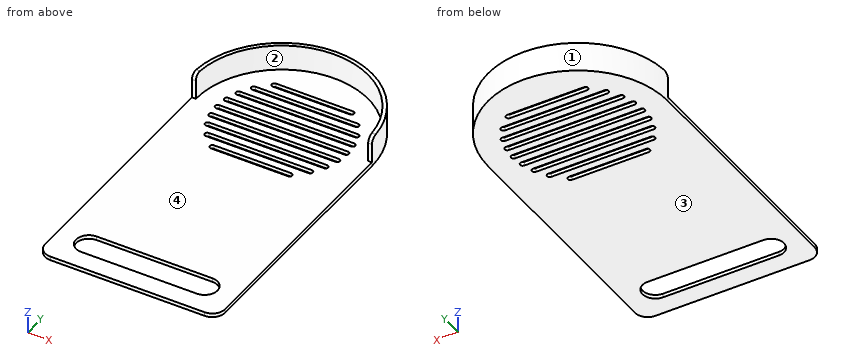
```python
from build123d import *

# Parameters (mm, degrees)
F1_DEPTH = 3
F2_DEPTH = 20
F3_R     = 5


with BuildPart() as f1:
    # F0 (on Top) → F1 (new body)
    with BuildSketch(Plane.XY):
        with BuildLine():
            Line((70, -190), (70, 0))
            Line((70, 0), (67, 0))
            ThreePointArc((67, 0), (0, 67), (-67, 0))
            Line((-67, 0), (-70, 0))
            Line((-70, 0), (-70, -190))
            ThreePointArc((-70, -190), (-67.071068, -197.071068), (-60, -200))
            Line((-60, -200), (60, -200))
            ThreePointArc((60, -200), (67.071068, -197.071068), (70, -190))
        make_face()
        with BuildLine():
            Line((45, -185), (-45, -185))
            ThreePointArc((-45, -185), (-55, -175), (-45, -165))
            Line((-45, -165), (45, -165))
            ThreePointArc((45, -165), (55, -175), (45, -185))
        make_face(mode=Mode.SUBTRACT)
        with BuildLine():
            ThreePointArc((30, -38), (32, -40), (30, -42))
            Line((30, -42), (-30, -42))
            ThreePointArc((-30, -42), (-32, -40), (-30, -38))
            Line((-30, -38), (30, -38))
        make_face(mode=Mode.SUBTRACT)
        with BuildLine():
            ThreePointArc((-40, -32), (-42, -30), (-40, -28))
            Line((-40, -28), (40, -28))
            ThreePointArc((40, -28), (42, -30), (40, -32))
            Line((40, -32), (-40, -32))
        make_face(mode=Mode.SUBTRACT)
        with BuildLine():
            ThreePointArc((45.825757, -18), (47.825757, -20), (45.825757, -22))
            Line((45.825757, -22), (-45.825757, -22))
            ThreePointArc((-45.825757, -22), (-47.825757, -20), (-45.825757, -18))
            Line((-45.825757, -18), (45.825757, -18))
        make_face(mode=Mode.SUBTRACT)
        with BuildLine():
            ThreePointArc((-48.989795, -12), (-50.989795, -10), (-48.989795, -8))
            Line((-48.989795, -8), (48.989795, -8))
            ThreePointArc((48.989795, -8), (50.989795, -10), (48.989795, -12))
            Line((48.989795, -12), (-48.989795, -12))
        make_face(mode=Mode.SUBTRACT)
        with BuildLine():
            Line((50, -2), (-50, -2))
            ThreePointArc((-50, -2), (-52, 0), (-50, 2))
            Line((-50, 2), (50, 2))
            ThreePointArc((50, 2), (52, 0), (50, -2))
        make_face(mode=Mode.SUBTRACT)
        with BuildLine():
            Line((48.989795, 8), (-48.989795, 8))
            ThreePointArc((-48.989795, 8), (-50.989795, 10), (-48.989795, 12))
            Line((-48.989795, 12), (48.989795, 12))
            ThreePointArc((48.989795, 12), (50.989795, 10), (48.989795, 8))
        make_face(mode=Mode.SUBTRACT)
        with BuildLine():
            Line((45.825757, 18), (-45.825757, 18))
            ThreePointArc((-45.825757, 18), (-47.825757, 20), (-45.825757, 22))
            Line((-45.825757, 22), (45.825757, 22))
            ThreePointArc((45.825757, 22), (47.825757, 20), (45.825757, 18))
        make_face(mode=Mode.SUBTRACT)
        with BuildLine():
            Line((40, 28), (-40, 28))
            ThreePointArc((-40, 28), (-42, 30), (-40, 32))
            Line((-40, 32), (40, 32))
            ThreePointArc((40, 32), (42, 30), (40, 28))
        make_face(mode=Mode.SUBTRACT)
        with BuildLine():
            Line((30, 38), (-30, 38))
            ThreePointArc((-30, 38), (-32, 40), (-30, 42))
            Line((-30, 42), (30, 42))
            ThreePointArc((30, 42), (32, 40), (30, 38))
        make_face(mode=Mode.SUBTRACT)
        with BuildLine():
            Line((67, 0), (70, 0))
            ThreePointArc((70, 0), (0, 70), (-70, 0))
            Line((-70, 0), (-67, 0))
            ThreePointArc((-67, 0), (0, 67), (67, 0))
        make_face()
    extrude(amount=-F1_DEPTH)

    # F0 (on Top) → F2 (join)
    with BuildSketch(Plane.XY):
        with BuildLine():
            Line((67, 0), (70, 0))
            ThreePointArc((70, 0), (0, 70), (-70, 0))
            Line((-70, 0), (-67, 0))
            ThreePointArc((-67, 0), (0, 67), (67, 0))
        make_face()
    extrude(amount=F2_DEPTH)

    # F3
    f3_edges = [f1.edges().sort_by_distance(p)[0] for p in [
        (-68.5, 0, 20),
        (68.5, 0, 20),
    ]]
    fillet(f3_edges, radius=F3_R)


solid = f1.part
```
Design review of the part built by this model. Coordinates are the model's own, in mm. Face numbers are marked on the shaded views. A direction names the side the tool comes from. Coordinates: 2 decimals unless noted, no trailing zeros. Write each loop counter-clockwise with the first axis right and the second up, starting at its lowest first coordinate (ties: lowest second). Pieces come first, ordered by that corner, then holes.
1) To check wall thickness, follow L1, parallel to Z at x = 35.5, y = -33.5; L2, parallel to Y at x = 2.5, z = 13.75; L3, parallel to X at y = 29.5, z = 16. State the ranges of each line that lie inside material, in increasing order.
2) Add section B-B (z = 5.25). Write out the cut boundary in (x, y), plus the area to 3 significant figures.
3) Mouldability with a two-part tool opening along Z and no side actions: class the marked faces 3 and 4 as +Z half, -Z half, draft (parallel to the pull), parting line (faces both ways), or undercut.
4) Add section C-C (x = -35). State how many separate pieces and enclosed holes the cut face has, plus the area to 3 significant figures.
5) Insertion check: pin 1 (2.5 mm diameter, centred on x = 68, z = 8, fed in from -Y); pin 2 (1.5 mm diameter, centred on x = -19.5, z = -1.5, fed in from +Y); pin 3 (12 mm diameter, centred on x = 45, z = 1.5, fed in from +Y). Each pin has a flat end and moves straight along its axis. Give the tip position at first contact, or say it passes through.
6) Machinability: for the marked faces 1 and 2, which of the approach directions +Z, -Z, +X, -X, +Y, -Y give a long, thin tool a straight path to every point of the face, cutting with its end or side? Answer none if there is none.
7) Add section D-D (y = -131). Write out the cut boundary in (x, z).
8) Add section A-A (y = -175). Write out the cut boundary in (x, z).
Check result:
1. L1: z = -3 to 0
1. L2: y = 66.95 to 69.96
1. L3: x = -63.48 to -60.16, 60.16 to 63.48
2. outline: (-70, 0) - (-67, 0) arc R67 cw to (67, 0) - (70, 0) arc R70 ccw to start
2. area: 646 mm2
3. face 3: -Z half
3. face 4: +Z half
4. separate pieces: 9
4. enclosed holes: 0
4. area: 708 mm2
5. pin 1: stops at y = 0
5. pin 2: stops at y = 67.44
5. pin 3: stops at y = 58.13
6. face 1: +Z, -Z, +Y
6. face 2: +Z, -Y
7. outline: (-70, -3) - (70, -3) - (70, 0) - (-70, 0) - close
8. outline: (-70, -3) - (-55, -3) - (-55, 0) - (-70, 0) - close; (55, -3) - (70, -3) - (70, 0) - (55, 0) - close
